```python
from build123d import *

# Parameters (mm, degrees)
F0_W     = 160
F0_H     = 320
F0_R     = 14
F0_R_2   = 3
F0_R_3   = 17.5
F1_DEPTH = 2.5


# Not quite as in the source:
# - a fillet or chamfer that OpenCascade refuses, or shapes differently, is made with other operations: its cross-section is extruded or revolved along the edge and cut away or added


with BuildPart() as f1:
    # F0 (on Front) → F1 (new body)
    with BuildSketch(Plane.XZ):
        with Locations((-1.8876045942, 29.6809725389)):
            Rectangle(F0_W, F0_H)
        with Locations((-31.8876045942, -60.3190274611)):
            Circle(F0_R, mode=Mode.SUBTRACT)
        with Locations((-1.8876045942, -95.3190274611)):
            Circle(F0_R_2, mode=Mode.SUBTRACT)
        with Locations((28.1123954058, -60.3190274611)):
            Circle(F0_R, mode=Mode.SUBTRACT)
        with Locations((-1.8876045942, -10.3190274611)):
            Circle(F0_R_3, mode=Mode.SUBTRACT)
        with Locations((-1.8876045942, 49.6809725389)):
            Circle(F0_R_3, mode=Mode.SUBTRACT)
        with Locations((-1.8876045942, 154.6809725389)):
            Circle(F0_R_2, mode=Mode.SUBTRACT)
    extrude(amount=F1_DEPTH)

    # F2: chamfer of 4 on 2 edges, made by hand

    # F2_s1 → F2_t2 (revolve, cut)
    with BuildSketch(Plane.XY.offset(154.6809725389)):
        Polygon((1.1123954058, 1.5), (5.1123954058, -2.5), (1.1123954058, -2.5), align=None)
    revolve(axis=Axis((-1.8876045942, -2.5, 154.6809725389), (0, -1, 0)), mode=Mode.SUBTRACT)

    # F2_s3 → F2_t4 (revolve, cut)
    with BuildSketch(Plane.XY.offset(-95.3190274611)):
        Polygon((1.1123954058, 1.5), (5.1123954058, -2.5), (1.1123954058, -2.5), align=None)
    revolve(axis=Axis((-1.8876045942, -2.5, -95.3190274611), (0, -1, 0)), mode=Mode.SUBTRACT)


solid = f1.part
```
Source: CAD feature listing. Evaluate the final solid. Frame: model axes, mm. Round coordinates to 2 decimals unless told otherwise and drop trailing zeros. Loops run counter-clockwise (first coordinate to the right, second up) from the corner with the lowest first, then second, coordinate; pieces in that order, holes last. Notation, with made-up numbers: M -40,66.5 L -21,66.5 A38 cw -21,105.5 Z; hole C 25.25,84.5 d5. An arc over 180 degrees is marked long. Use a Markdown table: item, result. Add a question column.
1. Cut plane A-A, the plane x = 27. Output: boundary loops of the cut face in (y, z).
2. Contact query for a flat-ended pin moving along its axis: pin 1 (21 mm diameter, centred on x = -1.89, z = 49.68, fed in from +Y). Output: stop coordinate, or through.
3. Ray query, line 1 along Z through (x, y) = (-14, -1.15); line 2 along X through (y, z) = (-0.95, -63); line 3 along X through (y, z) = (-1.35, 0.5). Return the intervals inside material, ascending. Write a range as [from, to].
4. Cut plane B-B, the plane z = -52. Output: boundary loops of the cut face in (x, y), and give its area (3 significant figures).
5. Pull-direction query (Z, two-part tool) for faces 1 (the conical face through (0.261, -0.156, -99.45)), 2 (the flat face through (-3, 0, 32)); classes: +Z half, -Z half, draft (parallel to the pull), parting line (faces both ways), or undercut.
6. Cut plane C-C, the plane y = -0.85. Output: boundary loops of the cut face in (x, z), and give its area (3 significant figures).
7. Cut plane D-D, the plane x = 11. Output: boundary loops of the cut face in (y, z), and give its area (3 significant figures).
Solution:
| question | item | result |
|---|---|---|
| 1 | outline | M -2.5,-130.32 L 0,-130.32 L 0,-74.27 L -2.5,-74.27 Z; M -2.5,-46.36 L 0,-46.36 L 0,189.68 L -2.5,189.68 Z |
| 2 | pin 1 | passes through |
| 3 | line 1 | z = [-130.32, -22.95], [2.31, 37.05], [62.31, 189.68] |
| 3 | line 2 | x = [-81.89, -45.63], [-18.15, 14.37], [41.85, 78.11] |
| 3 | line 3 | x = [-81.89, -15.64], [11.87, 78.11] |
| 4 | outline | M -81.89,-2.5 L -43.15,-2.5 L -43.15,0 L -81.89,0 Z; M -20.63,-2.5 L 16.85,-2.5 L 16.85,0 L -20.63,0 Z; M 39.37,-2.5 L 78.11,-2.5 L 78.11,0 L 39.37,0 Z |
| 4 | area | 287 mm2 |
| 5 | face 1 | undercut |
| 5 | face 2 | draft |
| 6 | outline | M -81.89,-130.32 L 78.11,-130.32 L 78.11,189.68 L -81.89,189.68 Z; hole C -31.89,-60.32 d28; hole C -1.89,-10.32 d35; hole C -1.89,49.68 d35; hole C -1.89,-95.32 d10.7; hole C -1.89,154.68 d10.7; hole C 28.11,-60.32 d28 |
| 6 | area | 47,900 mm2 |
| 7 | outline | M -2.5,-130.32 L 0,-130.32 L 0,-22.16 L -2.5,-22.16 Z; M -2.5,1.52 L 0,1.52 L 0,37.84 L -2.5,37.84 Z; M -2.5,61.52 L 0,61.52 L 0,189.68 L -2.5,189.68 Z |
| 7 | area | 682 mm2 |
